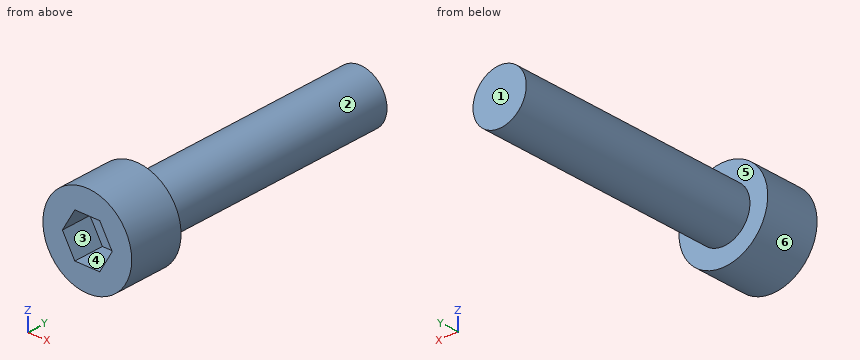
```python
from build123d import *

# Parameters (mm, degrees)
SKETCH1_R           = 2.8575
BOSS_EXTRUDE1_DEPTH = 3.5052
CUT_EXTRUDE1_DEPTH  = 1.9558
SKETCH3_R           = 1.7145
BOSS_EXTRUDE2_DEPTH = 15.875


with BuildPart() as part:
    # Sketch1 → Boss-Extrude1 (new body)
    with BuildSketch(Plane(origin=(0, 0, 0), x_dir=(1, 0, 0), z_dir=(0, 1, 0))):
        Circle(SKETCH1_R)
    extrude(amount=BOSS_EXTRUDE1_DEPTH)

    # Sketch2 → Cut-Extrude1 (cut)
    with BuildSketch(Plane.XZ):
        Polygon((1.603951217, 0), (0.801975608, 1.3890625), (-0.801975608, 1.3890625), (-1.603951217, 0), (-0.801975608, -1.3890625), (0.801975608, -1.3890625), align=None)
    extrude(amount=-CUT_EXTRUDE1_DEPTH, mode=Mode.SUBTRACT)

    # Sketch3 → Boss-Extrude2 (add)
    with BuildSketch(Plane(origin=(0, 3.5052, 0), x_dir=(1, 0, 0), z_dir=(0, 1, 0))):
        Circle(SKETCH3_R)
    extrude(amount=BOSS_EXTRUDE2_DEPTH)


solid = part.part
```
Input: part model. Units: mm. Frame: model coordinates. Face numbers are marked on the shaded views. A direction names the side the tool comes from. Give positions to 0.01 mm unless a question says otherwise; leave off trailing zeros. Loops run counter-clockwise (first coordinate to the right, second up) from the corner with the lowest first, then second, coordinate; pieces in that order, holes last.
1) Mould query, pull axis Z, two halves, no side actions, for the marked faces 1, 2 and 3. Classes: released by +Z, released by -Z, zero draft, split by the parting line, or undercut.
A:
face 1: zero draft
face 2: split by the parting line
face 3: undercut
2) Line query: L1, parallel to Z at x = -0.05, y = 9.5; L2, parallel to Y at x = 2.35, z = 0.65; L3, parallel to Y at x = -0.45, z = 0.6. Output: solid intervals per line, ascending.
A:
L1: z = -1.71 to 1.71
L2: y = 0 to 3.51
L3: y = 1.96 to 19.38
3) Section query D-D on x = 2.3. Return the cut outline in (y, z).
A:
outline: (0, -1.7) - (3.51, -1.7) - (3.51, 1.7) - (0, 1.7) - close
4) Section query C-C on z = 1.2. Return the cut outline in (x, y).
A:
outline: (-2.59, 0) - (-0.91, 0) - (-0.91, 1.96) - (0.91, 1.96) - (0.91, 0) - (2.59, 0) - (2.59, 3.51) - (1.22, 3.51) - (1.22, 19.38) - (-1.22, 19.38) - (-1.22, 3.51) - (-2.59, 3.51) - close
5) Reachability of the marked faces 4, 5 and 6 from +Z, -Z, +X, -X, +Y, -Y: full face, straight path, thin tool, end or side. Return the list, or none.
A:
face 4: -Y
face 5: +Y
face 6: +Y, -Y
6) Contact query for flat-ended pins moving along their axis: pin 1 (1.5 mm diameter, centred on y = 12, z = 0, fed in from -X); pin 2 (1.5 mm diameter, centred on x = -0.5, z = -1, fed in from -Y); pin 3 (1 mm diameter, centred on x = 0, y = 14.5, fed in from -Z); pin 4 (1.5 mm diameter, centred on x = 2, y = 8.5, fed in from +Z). Output: stop coordinate, or through.
A:
pin 1: stops at x = -1.71
pin 2: stops at y = 0
pin 3: stops at z = -1.71
pin 4: stops at z = 1.17
7) Section query B-B on y = 8.5. Return the cut outline in (x, z).
A:
outline: circle Ø3.43 at (0, 0)
8) Section query A-A on x = 0. Return the cut outline in (y, z).
A:
outline: (0, -2.86) - (3.51, -2.86) - (3.51, -1.71) - (19.38, -1.71) - (19.38, 1.71) - (3.51, 1.71) - (3.51, 2.86) - (0, 2.86) - (0, 1.39) - (1.96, 1.39) - (1.96, -1.39) - (0, -1.39) - close
